Verification items for the finished model (mm, model axes). Coordinates: 2 decimals unless noted, no trailing zeros. Loops run counter-clockwise (first coordinate to the right, second up) from the corner with the lowest first, then second, coordinate; pieces in that order, holes last. Notation, with made-up numbers: (48, -7.5) -> (103, -7.5) arc R4 ccw to (103, -3.5) -> close; hole circle Ø8 at (63, 27.5). An arc over 180 degrees is marked (long way). Write item = value, one per line.
Autodesk Inventor part; units mm, degrees
ref_plane "YZ Plane" through (0, 0, 0) normal (1, 0, 0) x (0, 1, 0)
ref_plane "XZ Plane" through (0, 0, 0) normal (0, 1, 0) x (-1, 0, 0)
ref_plane "XY Plane" through (0, 0, 0) normal (0, 0, 1) x (1, 0, 0)
sketch "Sketch1" plane through (0, 0, 0) normal (0, 1, 0) x (-1, 0, 0)
  line L0 (-100, 50) -> (100, 50)
  line L1 (100, 50) -> (100, -50)
  line L2 (100, -50) -> (-100, -50)
  line L3 (-100, -50) -> (-100, 50)
  line L4 (-100, 50) -> (100, -50) construction
  line L5 (100, 50) -> (-100, -50) construction
  point P0 (0, 0)
  dimension "d0" = 200
  dimension "d1" = 100
extrude "Extrusion1" add sketch "Sketch1" along normal blind 5
chamfer "Chamfer1" distance 15 angle 45 4 edges at (100, 2.5, -50) (100, 2.5, 50) (-100, 2.5, 50) (-100, 2.5, -50)
sketch "Sketch2" plane through (0, 5, 0) normal (0, 1, 0) x (1, 0, 0)
  line L0 (-85, -50) -> (85, -50)
  line L1 (85, 50) -> (85, -50)
  line L2 (85, 0) -> (0, 0)
  line L3 (85, 50) -> (-85, 50)
  line L4 (85, 0) -> (75, 0)
  line L5 (75, 0) -> (75, 50)
  line L6 (85, -50) -> (85, -45)
  line L7 (85, -45) -> (87.1749, -45)
  dimension "d7" = 10
  dimension "d15" = 5
hole "Hole2" at (85, 5, 45) direction (0, -1, 0) diameter 4.6 depth 12
pattern_linear "Rectangular Pattern1" count 10 spacing 10 along (0, 0, -1) of "Hole2"
mirror "Mirror1" about plane through (0, 0, 0) normal (1, 0, 0) of "Hole2", "Rectangular Pattern1"
sketch "Sketch4" plane through (0, 5, 0) normal (0, 1, 0) x (1, 0, 0)
  line L0 (-80.0603, -82.0418) -> (-80.0603, 17.9582)
  line L1 (90.6107, -82.0418) -> (90.6107, 17.9582)
  line L2 (-0.0013, -0.0056) -> (-0.0013, -50.0056)
  line L3 (83.0525, -0.0056) -> (83.0525, -82.0364)
  line L4 (83.0525, -0.0056) -> (-0.0013, -0.0056)
  line L5 (41.5256, -0.0056) -> (41.5256, -11.4056)
  line L6 (41.5256, -0.0056) -> (41.5256, 12.9944)
  line L7 (41.5256, 12.9944) -> (64.5256, 12.9944)
  line L8 (64.5256, 12.9944) -> (64.5256, -11.4056)
  line L9 (64.5256, -11.4056) -> (41.5256, -11.4056)
  line L10 (41.5256, -11.4056) -> (18.5256, -11.4056)
  line L11 (18.5256, -11.4056) -> (18.5256, 12.9944)
  line L12 (18.5256, 12.9944) -> (41.5256, 12.9944)
  line L13 (41.5256, 12.9944) -> (41.5256, 18.4944)
  line L14 (41.5256, 18.4944) -> (64.5256, 18.4944)
  line L15 (64.5256, 18.4944) -> (64.5256, 12.9944)
  line L16 (41.5256, 18.4944) -> (18.5256, 18.4944)
  line L17 (18.5256, 12.9944) -> (18.5256, 18.4944)
  line L18 (41.5256, -11.4056) -> (41.5256, -16.5056)
  line L19 (41.5256, -16.5056) -> (64.5256, -16.5056)
  line L20 (64.5256, -16.5056) -> (64.5256, -11.4056)
  line L21 (41.5256, -16.5056) -> (18.5256, -16.5056)
  line L22 (18.5256, -16.5056) -> (18.5256, -11.4056)
  point P0 (0, 0)
  dimension "d31" = 100
  dimension "d32" = 50
  dimension "d35" = 23
  dimension "d36" = 23
  dimension "d37" = 5.5
  dimension "d38" = 23
  dimension "d39" = 23
  dimension "d40" = 5.1
  dimension "d41" = 23
  dimension "d42" = 23
  dimension "d56" = 35
extrude "Extrusion3" cut sketch "Sketch4" against normal blind 10 contours L7 L13 L14 L15 | L20 L19 L18 L9 | L18 L21 L22 L10 | L12 L17 L16 L13
sketch "Sketch6" plane through (0, 0, 0) normal (0, -1, 0) x (1, 0, 0)
  line L0 (100, 35) -> (100, -35)
  line L1 (100, 0) -> (-99.9985, 0)
  line L2 (0, 0) -> (-99.9985, 0)
  line L3 (-49.9993, 0) -> (-49.9993, 50)
  line L4 (-85, 50) -> (85, 50)
  line L5 (-49.9993, 0) -> (-49.9993, -50.9458)
  circle A0 centre (-50.1056, -13.7921) radius 1.5
  dimension "d70" = 3
hole "Hole3" at (-50.1056, 0, -13.7921) direction (0, 1, 0) diameter 3 depth 12.7625
pattern_linear "Rectangular Pattern2" count 3 spacing 5 along (1, 0, 0) count 3 spacing 10 along (-1, 0, 0) of "Hole3"
mirror "Mirror2" about plane through (0, 0, 0) normal (0, 0, 1) of "Hole3", "Rectangular Pattern2"
sketch "Sketch7" plane through (0, 5, 0) normal (0, 1, 0) x (1, 0, 0)
  circle A0 centre (-85, -45) radius 2.3
  line L0 (-85, -45) -> (-75, -45)
  circle A1 centre (-75, -45) radius 2.3
  point P0 (0, 0)
  dimension "d84" = 10
  dimension "d85" = 4.6
hole "Hole4" at (-75, 5, 45) direction (0, -1, 0) diameter 4.6 depth 7
pattern_linear "Rectangular Pattern3" count 16 spacing 10 along (1, 0, 0) of "Hole4"
mirror "Mirror3" about plane through (0, 0, 0) normal (0, 0, 1) of "Hole4", "Rectangular Pattern3"
sketch "Sketch8" plane through (0, 5, 0) normal (0, 1, 0) x (1, 0, 0)
  line L0 (-6.2494, -15) -> (-36.2494, -15)
  line L1 (-36.2494, -15) -> (-36.2494, 15)
  line L2 (-36.2494, 15) -> (-6.2494, 15)
  line L3 (-6.2494, 15) -> (-6.2494, -15)
  line L4 (-6.2494, -15) -> (-36.2494, 15) construction
  line L5 (-36.2494, -15) -> (-6.2494, 15) construction
  point P0 (0, 0)
  point P1 (-21.2494, 0)
  dimension "d96" = 30
  dimension "d97" = 30
extrude "Extrusion5" cut sketch "Sketch8" against normal blind 10
properties part number "Chasis1"
1) Sectioned sample at A-A, the plane z = -5. Record the cut outline in (x, y).
Ans:
outline = (-100, 0) -> (-87.3, 0) -> (-87.3, 5) -> (-100, 5) -> close; (-82.7, 0) -> (-36.25, 0) -> (-36.25, 5) -> (-82.7, 5) -> close; (-6.25, 0) -> (82.7, 0) -> (82.7, 5) -> (-6.25, 5) -> close; (87.3, 0) -> (100, 0) -> (100, 5) -> (87.3, 5) -> close
2) Sectioned sample at C-C, the plane x = 75. Record the cut outline in (y, z), plus the area to 3 significant figures.
Ans:
outline = (0, -50) -> (5, -50) -> (5, -47.3) -> (0, -47.3) -> close; (0, -42.7) -> (5, -42.7) -> (5, 42.7) -> (0, 42.7) -> close; (0, 47.3) -> (5, 47.3) -> (5, 50) -> (0, 50) -> close
area = 454 mm2
3) Material ranges on line 1 (X direction, y = 2.1, z = 5); line 2 (Z direction, x = 5, y = 3); line 3 (Z direction, x = -55, y = 3.2), recorded low to high.
Ans:
line_1 = -100 to -87.3, -82.7 to -36.25, -6.25 to 82.7, 87.3 to 100
line_2 = -50 to -47.3, -42.7 to 42.7, 47.3 to 50
line_3 = -50 to -47.3, -42.7 to -15.29, -12.3 to 12.3, 15.29 to 42.7, 47.3 to 50
4) Release check for a two-part mould opening along Z. For faces 1 (the face through (-1, 2, -50)), 2 (the face through (-27.04, 2.46, -46.06)), 3 (the face through (-93, 2, 42)) record: pulls with the +Z half, pulls with the -Z half, needs draft (parallel to the pull), parting line crosses it, or undercut.
Ans:
face_1 = pulls with the -Z half
face_2 = undercut
face_3 = pulls with the +Z half
5) Sectioned sample at D-D, the plane z = 25. Record the cut outline in (x, y).
Ans:
outline = (-100, 0) -> (-87.3, 0) -> (-87.3, 5) -> (-100, 5) -> close; (-82.7, 0) -> (82.7, 0) -> (82.7, 5) -> (-82.7, 5) -> close; (87.3, 0) -> (100, 0) -> (100, 5) -> (87.3, 5) -> close
6) Sectioned sample at B-B, the plane x = 35. Record the cut outline in (y, z), plus the area to 3 significant figures.
Ans:
outline = (0, -50) -> (5, -50) -> (5, -47.3) -> (0, -47.3) -> close; (0, -42.7) -> (5, -42.7) -> (5, -18.49) -> (0, -18.49) -> close; (0, -12.99) -> (5, -12.99) -> (5, 11.41) -> (0, 11.41) -> close; (0, 16.51) -> (5, 16.51) -> (5, 42.7) -> (0, 42.7) -> close; (0, 47.3) -> (5, 47.3) -> (5, 50) -> (0, 50) -> close
area = 401 mm2
